Verification items for the finished model (mm, model axes). Face numbers are marked on the shaded views. A direction names the side the tool comes from. Coordinates: 2 decimals unless noted, no trailing zeros. Order: outer loops, then holes, each group sorted by start corner. A loop starts at its lowest first (then second) coordinate and runs counter-clockwise, first axis right, second up. Notation, with made-up numbers: M -12,-26 L 35,-26 A24 ccw 35,5 Z; hole C 81,53.25 d3. An arc over 180 degrees is marked long. Return JSON: item names as keys, results as strings. Group by question number.
Q1. Thickness scan on probe 1 along Z at (x, y) = (-37.3, 17.5); probe 2 along Z at (x, y) = (-22, 9.5); probe 3 along Y at (x, z) = (-15, 67). Record the ranges inside material, lowest first.
Q2. Go/stop test with flat-tipped pins: pin 1 Ø2.5 at (x, z) = (-23, 67.5) entering from -Y; pin 2 Ø10 at (x, z) = (24, 47) entering from -Y; pin 3 Ø6 at (y, z) = (-16.5, 44) entering from +X. Record where each tip stops, or that it passes through.
Q3. Mould release check, pull along Y, two halves, no side actions. Record for the marked faces 4, 5, 6 and 7: pulls with the +Y half, pulls with the -Y half, needs draft (parallel to the pull), parting line crosses it, or undercut.
Q4. Section check D-D, the plane y = 25.5. Enter the section's corners in (x, z), then the cut area to 3 significant figures.
Q5. Section check C-C, the plane z = 40. Enter the section's corners in (x, y), then the cut area to 3 significant figures.
Q6. Access from +Z, -Z, +X, -X, +Y, -Y to the whole of each face (thin tool, end or side, straight path). Record for the marked faces 1, 2 and 3.
Q7. Section check B-B, the plane y = 4. Enter the section's corners in (x, z), then the cut area to 3 significant figures.
Q8. Section check A-A, the plane x = 5.5. Enter the section's corners in (y, z), then the cut area to 3 significant figures.
from build123d import *

# Parameters (mm, degrees)
SKETCH_W        = 76
SKETCH_H        = 76
SKETCH_R        = 35
SKETCH_R_2      = 1.7
PAD_DEPTH       = 65.3
SKETCH001_R     = 60
SKETCH001_R_2   = 38
POCKET_DEPTH    = 61.3
SKETCH002_R     = 38
PAD001_DEPTH    = 3
SKETCH003_W     = 100
SKETCH003_H     = 100
SKETCH003_W_2   = 80
SKETCH003_H_2   = 68
POCKET001_DEPTH = 68.301
SKETCH004_W     = 68
SKETCH004_H     = 16
PAD002_DEPTH    = 22
POCKET002_DEPTH = 25
POCKET003_DEPTH = 20
SKETCH030_R     = 35
POCKET004_DEPTH = 18
SKETCH031_R     = 1.7
POCKET005_DEPTH = 30
SKETCH022_R     = 7
SKETCH022_R_2   = 1.5
SKETCH022_R_3   = 2.2
SKETCH022_W     = 3.5
SKETCH022_H     = 5
POCKET006_DEPTH = 5
SKETCH032_W     = 220
SKETCH032_H     = 220
POCKET007_DEPTH = 68.301
POCKET008_DEPTH = 20


with BuildPart() as part:
    # Sketch → Pad (new body)
    with BuildSketch(Plane.XY):
        Rectangle(SKETCH_W, SKETCH_H)
        Circle(SKETCH_R, mode=Mode.SUBTRACT)
        with Locations((-30, 30)):
            Circle(SKETCH_R_2, mode=Mode.SUBTRACT)
        with Locations((30, 30)):
            Circle(SKETCH_R_2, mode=Mode.SUBTRACT)
        with Locations((30, -30)):
            Circle(SKETCH_R_2, mode=Mode.SUBTRACT)
        with Locations((-30, -30)):
            Circle(SKETCH_R_2, mode=Mode.SUBTRACT)
    extrude(amount=PAD_DEPTH)

    # Sketch001 → Pocket (cut)
    with BuildSketch(Plane.XY.offset(65.3)):
        Circle(SKETCH001_R)
        Circle(SKETCH001_R_2, mode=Mode.SUBTRACT)
    extrude(amount=-POCKET_DEPTH, mode=Mode.SUBTRACT)

    # Sketch002 → Pad001 (new body)
    with BuildSketch(Plane.XY.offset(65.3)):
        Circle(SKETCH002_R)
    extrude(amount=PAD001_DEPTH)

    # Sketch003 → Pocket001 (cut, through all)
    with BuildSketch(Plane.XY.offset(68.3)):
        Rectangle(SKETCH003_W, SKETCH003_H)
        Rectangle(SKETCH003_W_2, SKETCH003_H_2, mode=Mode.SUBTRACT)
    extrude(amount=-POCKET001_DEPTH, mode=Mode.SUBTRACT)

    # Sketch004 → Pad002 (new body)
    with BuildSketch(Plane(origin=(-38, 0, 0), x_dir=(0, -1, 0), z_dir=(-1, 0, 0))):
        with Locations((0, 44)):
            Rectangle(SKETCH004_W, SKETCH004_H)
    extrude(amount=-PAD002_DEPTH)

    # Sketch005 → Pocket002 (cut)
    with BuildSketch(Plane(origin=(0, 0, 36), x_dir=(1, 0, 0), z_dir=(0, 0, -1))):
        Polygon((-38, 23), (-38, -23), (-24, -34), (-55, -34), (-55, 34), (-24, 34), align=None)
    extrude(amount=-POCKET002_DEPTH, mode=Mode.SUBTRACT)

    # Sketch029 → Pocket003 (cut)
    with BuildSketch(Plane.YZ.offset(-16)):
        Polygon((-15.883419, 41.2), (-14.266838, 44), (-15.883419, 46.8), (-19.116581, 46.8), (-20.733162, 44), (-19.116581, 41.2), align=None)
        Polygon((14.266838, 44), (15.883419, 41.2), (19.116581, 41.2), (20.733162, 44), (19.116581, 46.8), (15.883419, 46.8), align=None)
    extrude(amount=-POCKET003_DEPTH, mode=Mode.SUBTRACT)

    # Sketch030 → Pocket004 (cut)
    with BuildSketch(Plane.XY.offset(52)):
        Circle(SKETCH030_R)
    extrude(amount=-POCKET004_DEPTH, mode=Mode.SUBTRACT)

    # Sketch031 → Pocket005 (cut)
    with BuildSketch(Plane(origin=(-38, 0, 0), x_dir=(0, -1, 0), z_dir=(-1, 0, 0))):
        with Locations((-17.5, 44)):
            Circle(SKETCH031_R)
        with Locations((17.5, 44)):
            Circle(SKETCH031_R)
        with BuildLine():
            ThreePointArc((-5, 51), (-12, 44), (-5, 37))
            Line((-5, 37), (5, 37))
            ThreePointArc((5, 37), (12, 44), (5, 51))
            Line((-5, 51), (5, 51))
        make_face()
    extrude(amount=-POCKET005_DEPTH, mode=Mode.SUBTRACT)

    # Sketch022 → Pocket006 (cut)
    with BuildSketch(Plane.XY.offset(68.3)):
        Circle(SKETCH022_R)
        with Locations((-27, 0)):
            Circle(SKETCH022_R_2)
        with Locations((0, -15)):
            Circle(SKETCH022_R_3)
        with Locations((0, 15)):
            Circle(SKETCH022_R_3)
        with Locations((15, 0)):
            Circle(SKETCH022_R_3)
        with Locations((-15, 0)):
            Circle(SKETCH022_R_3)
        with BuildLine():
            ThreePointArc((-23.514078, 16.973159), (-22.611882, 11.388713), (-17.027436, 12.290908))
            ThreePointArc((-12.290908, 17.027436), (-14.849242, 14.849242), (-17.027436, 12.290908))
            ThreePointArc((-12.290908, 17.027436), (-11.388713, 22.611882), (-16.973159, 23.514078))
            ThreePointArc((-16.973159, 23.514078), (-20.506097, 20.506097), (-23.514078, 16.973159))
        make_face()
        with BuildLine():
            ThreePointArc((12.290908, -17.027436), (14.849242, -14.849242), (17.027436, -12.290908))
            ThreePointArc((23.514078, -16.973159), (22.611882, -11.388713), (17.027436, -12.290908))
            ThreePointArc((16.973159, -23.514078), (20.506097, -20.506097), (23.514078, -16.973159))
            ThreePointArc((12.290908, -17.027436), (11.388713, -22.611882), (16.973159, -23.514078))
        make_face()
        with BuildLine():
            ThreePointArc((23.514078, 16.973159), (20.506097, 20.506097), (16.973159, 23.514078))
            ThreePointArc((16.973159, 23.514078), (11.388713, 22.611882), (12.290908, 17.027436))
            ThreePointArc((17.027436, 12.290908), (14.849242, 14.849242), (12.290908, 17.027436))
            ThreePointArc((17.027436, 12.290908), (22.611882, 11.388713), (23.514078, 16.973159))
        make_face()
        with BuildLine():
            ThreePointArc((-16.973159, -23.514078), (-11.388713, -22.611882), (-12.290908, -17.027436))
            ThreePointArc((-17.027436, -12.290908), (-14.849242, -14.849242), (-12.290908, -17.027436))
            ThreePointArc((-17.027436, -12.290908), (-22.611882, -11.388713), (-23.514078, -16.973159))
            ThreePointArc((-23.514078, -16.973159), (-20.506097, -20.506097), (-16.973159, -23.514078))
        make_face()
        with Locations((-22.25, 0)):
            Rectangle(SKETCH022_W, SKETCH022_H)
    extrude(amount=-POCKET006_DEPTH, mode=Mode.SUBTRACT)

    # Sketch032 → Pocket007 (cut, through all)
    with BuildSketch(Plane.XY.offset(68.3)):
        Rectangle(SKETCH032_W, SKETCH032_H)
        Polygon((-67.882251, 0), (0, 67.882251), (67.882251, 0), (0, -67.882251), align=None, mode=Mode.SUBTRACT)
    extrude(amount=-POCKET007_DEPTH, mode=Mode.SUBTRACT)

    # Sketch033 → Pocket008 (cut)
    with BuildSketch(Plane(origin=(33.941125, 33.941125, 0), x_dir=(-0.707107, 0.707107, 0), z_dir=(0.707107, 0.707107, 0))):
        with BuildLine():
            ThreePointArc((-6, 65), (-11, 60), (-6, 55))
            Line((-6, 55), (6, 55))
            ThreePointArc((6, 55), (11, 60), (6, 65))
            Line((-6, 65), (6, 65))
        make_face()
    extrude(amount=-POCKET008_DEPTH, mode=Mode.SUBTRACT)


solid = part.part
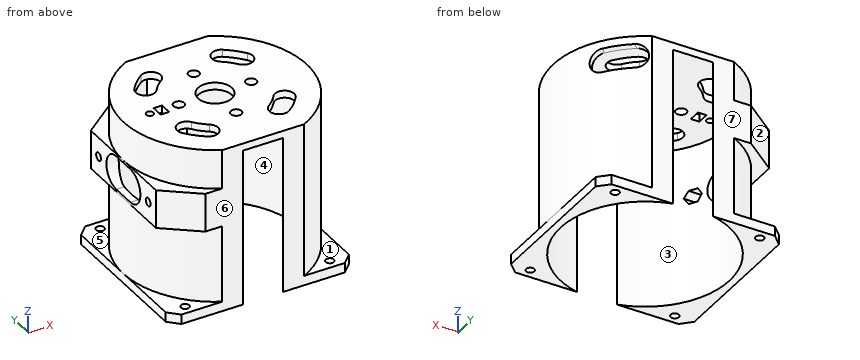
Numbers:
{
 "1": {"probe 1": "z = 0 to 4, 36 to 42.3, 45.7 to 52", "probe 2": "z = 65.3 to 68.3", "probe 3": "y = -34 to -24.25, -14.7 to -2.2, 2.2 to 14.7, 24.25 to 34"},
 "2": {"pin 1": "stops at y = -31.16", "pin 2": "stops at y = -32.91", "pin 3": "stops at x = 35.52"},
 "3": {"face 4": "undercut", "face 5": "needs draft", "face 6": "pulls with the -Y half", "face 7": "pulls with the +Y half"},
 "4": {"outline": "M -38,0 L -23.97,0 L -23.97,65.3 L 23.97,65.3 L 23.97,65 L 28.17,65 L 28.17,68.3 L -28.17,68.3 L -28.17,52 L -34.82,52 L -34.82,36 L -28.17,36 L -28.17,4 L -38,4 Z; M 23.97,0 L 38,0 L 38,4 L 28.17,4 L 28.17,55 L 23.97,55 Z", "area": "860 mm2"},
 "5": {"outline": "M -38,-23 L -24,-34 L -8.31,-34 A35 cw -33.31,-10.74 L -38,-10.74 Z; M -38,10.74 L -33.31,10.74 A35 cw -8.31,34 L -24,34 L -38,23 Z; M 8.31,-34 L 16.97,-34 A38 ccw 16.97,34 L 8.31,34 A35 cw Z", "area": "704 mm2"},
 "6": {"face 1": "+Z, +X, -Y", "face 2": "+Z, -X, +Y", "face 3": "-Z"},
 "7": {"outline": "M -38,0 L -34.77,0 L -34.77,37 L -38,37 L -38,36 L -37.79,36 L -37.79,4 L -38,4 Z; M -38,51 L -34.77,51 L -34.77,65.3 L -5.74,65.3 L -5.74,68.3 L -37.79,68.3 L -37.79,52 L -38,52 Z; M 5.74,65.3 L 34.77,65.3 L 34.77,0 L 38,0 L 38,4 L 37.79,4 L 37.79,68.3 L 5.74,68.3 Z", "area": "546 mm2"},
 "8": {"outline": "M -34,65.3 L -4.33,65.3 L -4.33,68.3 L -34,68.3 Z; M 4.33,65.3 L 34,65.3 L 34,68.3 L 4.33,68.3 Z", "area": "178 mm2"}
}
